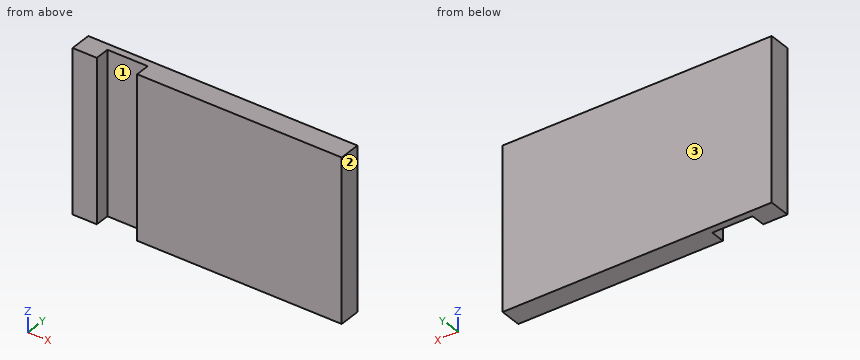
```python
from build123d import *

# Parameters (mm, degrees)
F0_W     = 127
F0_H     = 76.2
F1_DEPTH = 10.16
F2_W     = 19.05
F2_H     = 6.0776587872
F3_DEPTH = 25.4
F4_DEPTH = 25.4
F5_DEPTH = 50.8
F6_W     = 19.05
F6_H     = 6.8539392034
F7_DEPTH = 127


with BuildPart() as f1:
    # F0 (on Front) → F1 (new body)
    with BuildSketch(Plane.XZ):
        with Locations((-63.5, 38.1)):
            Rectangle(F0_W, F0_H)
    extrude(amount=F1_DEPTH)

    # F2 (on face) → F3 (cut)
    with BuildSketch(Plane.XY.offset(76.2)):
        with Locations((-103.3981527448, -7.1211706064)):
            Rectangle(F2_W, F2_H)
    extrude(amount=-F3_DEPTH, mode=Mode.SUBTRACT)

    # F4 (cut): a face of the model
    f4_faces = [f1.faces().sort_by_distance(p)[0] for p in [
        (-103.3981527448, -7.1211706064, 50.8),
    ]]
    extrude(f4_faces, amount=-F4_DEPTH, mode=Mode.SUBTRACT)

    # F5 (add): a face of the model
    f5_faces = [f1.faces().sort_by_distance(p)[0] for p in [
        (-103.3981527448, -7.1211706064, 25.4),
    ]]
    extrude(f5_faces, amount=F5_DEPTH)

    # F6 (on face) → F7 (cut)
    with BuildSketch(Plane.XY.offset(76.2)):
        with Locations((-106.0485850334, -6.7330303983)):
            Rectangle(F6_W, F6_H)
    extrude(amount=-F7_DEPTH, mode=Mode.SUBTRACT)


solid = f1.part
```
Geometry check sheet. Reference: the model listing, model coordinates, mm. Face numbers are marked on the shaded views. Coordinates: 2 decimals unless noted, no trailing zeros. Loops run counter-clockwise (first coordinate to the right, second up) from the corner with the lowest first, then second, coordinate; pieces in that order, holes last.
Item 1: Go/stop test with flat-tipped pins: pin 1 Ø5.5 at (x, z) = (-103.5, 40.5) entering from -Y; pin 2 Ø2 at (x, y) = (-109.5, -5) entering from -Z. Record where each tip stops, or that it passes through.
Item 2: Sectioned sample at C-C, the plane x = -107.5. Record the boundary of the cut face in (y, z).
Item 3: Release check for a two-part mould opening along X. For the marked faces 1, 2 and 3 record: released by +X, released by -X, zero draft, split by the parting line, or undercut.
Item 4: Sectioned sample at B-B, the plane z = 45. Record the boundary of the cut face in (x, y), then the cut area to 3 significant figures.
Item 5: Thickness scan on line 1 (X direction, y = -7.75, z = 13); line 2 (Y direction, x = -114, z = 59). Record the ranges inside material, lowest first.
Item 6: Sectioned sample at A-A, the plane y = -6. Record the boundary of the cut face in (x, z).
Check result:
1. pin 1: stops at y = -3.31
1. pin 2: passes through
2. outline: (-3.31, 0) - (0, 0) - (0, 76.2) - (-3.31, 76.2) - close
3. face 1: undercut
3. face 2: released by +X
3. face 3: zero draft
4. outline: (-127, -10.16) - (-115.57, -10.16) - (-115.57, -3.31) - (-96.52, -3.31) - (-96.52, -10.16) - (0, -10.16) - (0, 0) - (-127, 0) - close
4. area: 1,160 mm2
5. line 1: x = -127 to -115.57, -96.52 to 0
5. line 2: y = -3.31 to 0
6. outline: (-127, 0) - (-115.57, 0) - (-115.57, 76.2) - (-127, 76.2) - close; (-96.52, 0) - (0, 0) - (0, 76.2) - (-96.52, 76.2) - close
